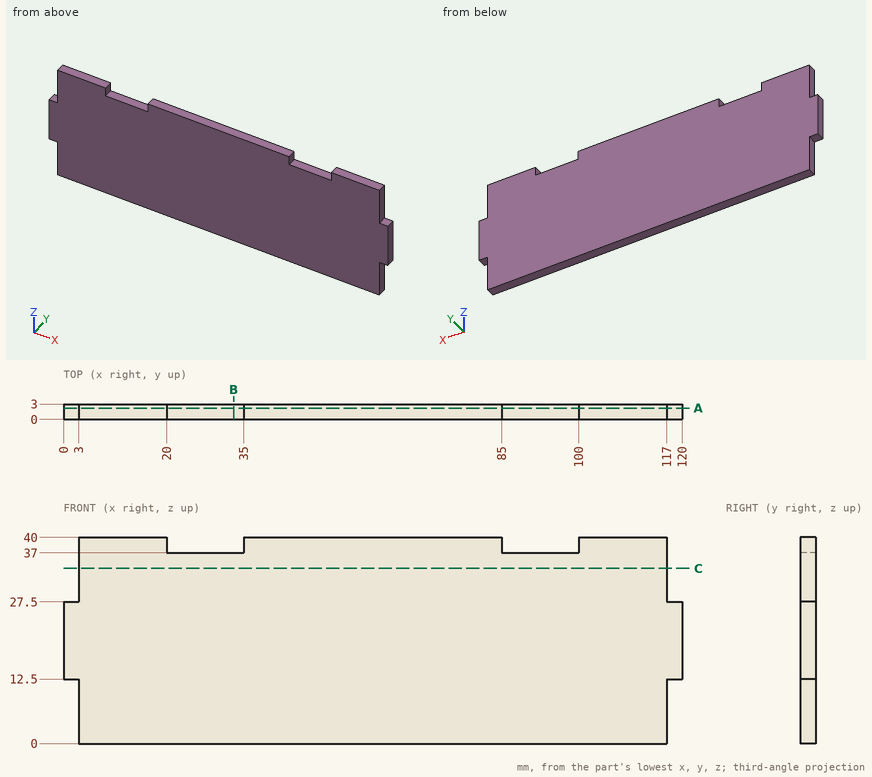
For this review, use the dimensioned drawing (mm, ordinates from the lowest corner) and the shaded views. Round coordinates to 2 decimals unless told otherwise and drop trailing zeros. Write each loop counter-clockwise with the first axis right and the second up, starting at its lowest first coordinate (ties: lowest second). Pieces come first, ordered by that corner, then holes. Notation, with made-up numbers: (49, 61.25) - (73, 61.25) arc R14 cw to (73, 72.25) - close; hole circle Ø5 at (19, 41.25). An arc over 180 degrees is marked (long way). Answer as a JSON object with one key per item and string values.
1. We need section B-B on x = 33. Give the boundary of the cut face in (y, z).
Response values:
{"outline": "(0, 0) - (3, 0) - (3, 37) - (0, 37) - close"}
2. To check wall thickness, follow line 1 along X through (y, z) = (0.5, 3); line 2 along Z through (x, y) = (86, 0.7). State the ranges of each line that lie inside material, in increasing order.
Response values:
{"line 1": "x = 3 to 117", "line 2": "z = 0 to 37"}
3. We need section C-C on z = 34. Give the boundary of the cut face in (x, y), then the cut area to 3 significant figures.
Response values:
{"outline": "(3, 0) - (117, 0) - (117, 3) - (3, 3) - close", "area": "342 mm2"}
4. We need section A-A on y = 2.2. Give the boundary of the cut face in (x, z).
Response values:
{"outline": "(0, 12.5) - (3, 12.5) - (3, 0) - (117, 0) - (117, 12.5) - (120, 12.5) - (120, 27.5) - (117, 27.5) - (117, 40) - (100, 40) - (100, 37) - (85, 37) - (85, 40) - (35, 40) - (35, 37) - (20, 37) - (20, 40) - (3, 40) - (3, 27.5) - (0, 27.5) - close"}
5. For pin 1 Ø1.5 at (x, y) = (90.5, 1) entering from +Z; pin 2 Ø0.9 at (y, z) = (2, 3.5) entering from -X; pin 3 Ø1.5 at (y, z) = (2, 39) entering from +X, all flat-tipped, find the tip position at first contact; note any pin that passes through.
Response values:
{"pin 1": "stops at z = 37", "pin 2": "stops at x = 3", "pin 3": "stops at x = 117"}
